Can you work these out from the drawing? Everything is in mm from the part's minimum corner. Coordinates: 2 decimals unless noted, no trailing zeros. Loops run counter-clockwise (first coordinate to the right, second up) from the corner with the lowest first, then second, coordinate; pieces in that order, holes last. Notation, with made-up numbers: M -33,30.5 L 10,30.5 A27 ccw 10,68.5 Z; hole C 65.5,87.5 d11. An arc over 180 degrees is marked long. Write each question's results on one line, items separated by ' | '.
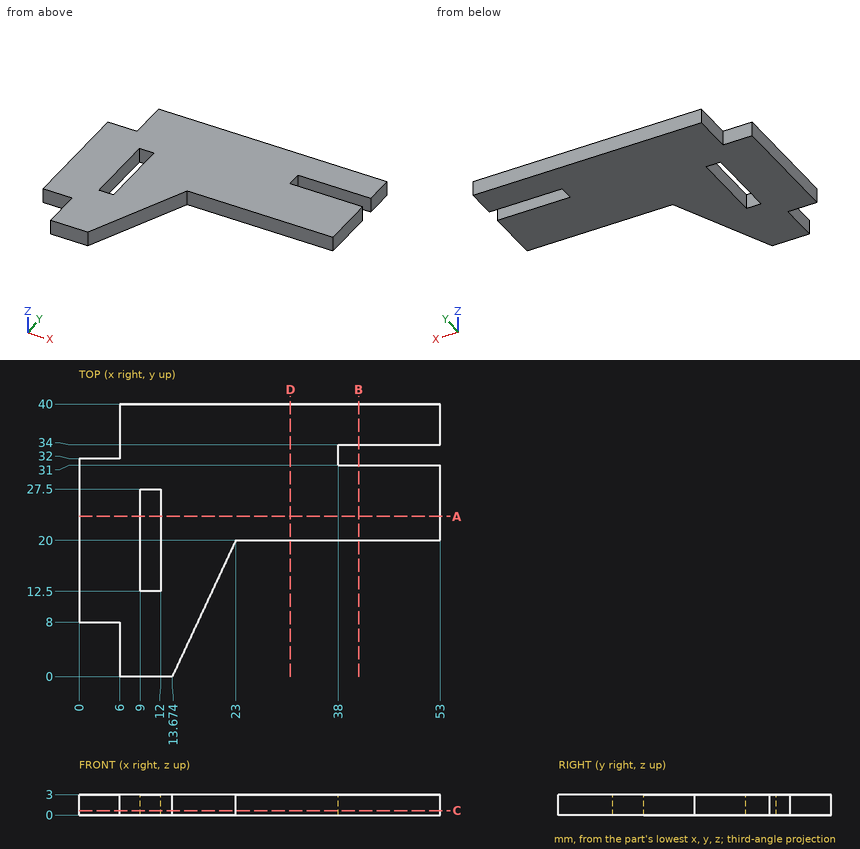
(1) Will these pins go through, and if not, where does the flat tip stop? P1, Ø12, axis at x = 13.5, y = 34.5, coming from the -Z side; P2, Ø0.9, axis at y = 5, z = 1.5, coming from the -X side; P3, Ø1.5, axis at x = 31, z = 1.5, coming from the -Y side.
Reported:
P1: stops at z = 0 | P2: stops at x = 6 | P3: stops at y = 20
(2) Imagine slicing it at B-B, the plane x = 41. List the corners of the cut face in (y, z) for me, and give its area (3 significant figures).
Reported:
outline: M 20,0 L 31,0 L 31,3 L 20,3 Z; M 34,0 L 40,0 L 40,3 L 34,3 Z | area: 51.0 mm2
(3) Imagine slicing it at A-A, the plane y = 23.5. List the corners of the cut face in (x, z) for me, and give its area (3 significant figures).
Reported:
outline: M 0,0 L 9,0 L 9,3 L 0,3 Z; M 12,0 L 53,0 L 53,3 L 12,3 Z | area: 150 mm2
(4) Imagine slicing it at C-C, the plane z = 0.65. List the corners of the cut face in (x, y) for me.
Reported:
outline: M 0,8 L 6,8 L 6,0 L 13.67,0 L 23,20 L 53,20 L 53,31 L 38,31 L 38,34 L 53,34 L 53,40 L 6,40 L 6,32 L 0,32 Z; hole M 9,12.5 L 12,12.5 L 12,27.5 L 9,27.5 Z
(5) Imagine slicing it at D-D, the plane x = 31. List the corners of the cut face in (y, z) for me, and give its area (3 significant figures).
Reported:
outline: M 20,0 L 40,0 L 40,3 L 20,3 Z | area: 60.0 mm2
(6) Please list where these lines run through material, in increasing order: probe 1 along X at (y, z) = (24.5, 0.45); probe 2 along X at (y, z) = (38, 1.5); probe 3 along Y at (x, z) = (44, 2.85). Write a range as from..to.
Reported:
probe 1: x = 0..9, 12..53 | probe 2: x = 6..53 | probe 3: y = 20..31, 34..40
